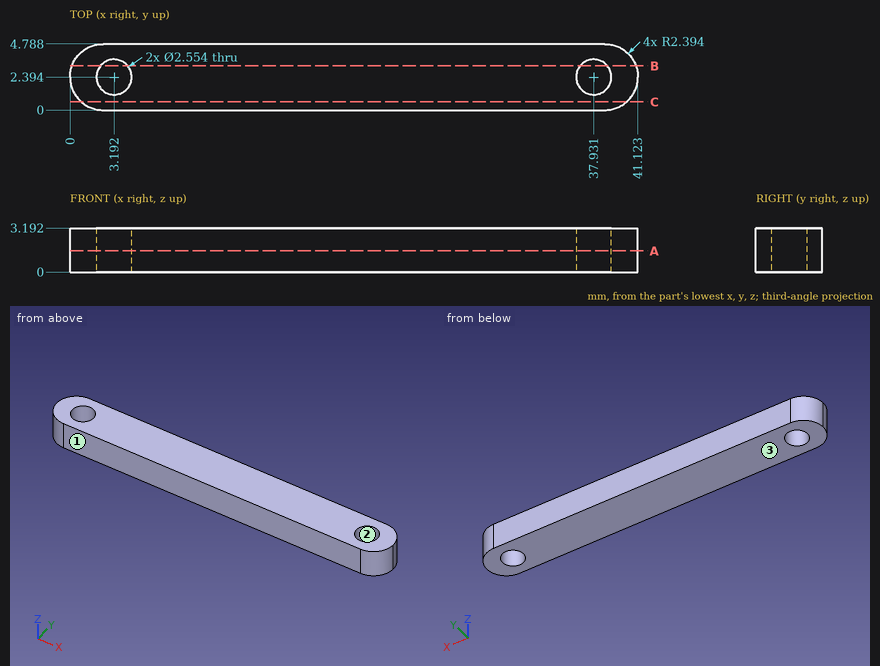
Verification items for this drawing (mm, ordinates from the low corner). Give positions to 0.01 mm unless a question says otherwise; leave off trailing zeros. Loops run counter-clockwise (first coordinate to the right, second up) from the corner with the lowest first, then second, coordinate; pieces in that order, holes last. Notation, with made-up numbers: M 84,14 L 119,14 A35 ccw 119,49 Z; hole C 59.25,20.25 d4. An arc over 180 degrees is marked long. Answer as a JSON object with one key per item and string values. Group by question number.
Q1. Material ranges on line 1 along X through (y, z) = (2.7, 2.65); line 2 along X through (y, z) = (2.6, 2.8); line 3 along Y through (x, z) = (37, 2.65) (1 decimal), recorded low to high. Write a range as [from, to].
Q2. Cross-section at A-A on z = 1.55. Give the number of separate pieces and of enclosed holes in the cut face, then the cut area to 3 significant figures.
Q3. Cross-section at B-B on y = 3.2. Record the cut outline in (x, z).
Q4. Cross-section at C-C on y = 0.6. Record the cut outline in (x, z).
Q5. Release check for a two-part mould opening along Y. For the marked faces 1, 2 and 3 record: released by +Y, released by -Y, zero draft, split by the parting line, or undercut.
Evaluation:
{
 "1": {"line 1": "x = [0.02, 1.95], [4.43, 36.69], [39.17, 41.1]", "line 2": "x = [0.01, 1.93], [4.45, 36.67], [39.19, 41.11]", "line 3": "y = [0, 1.5], [3.3, 4.8]"},
 "2": {"separate pieces": "1", "enclosed holes": "2", "area": "182 mm2"},
 "3": {"outline": "M 0.14,0 L 2.2,0 L 2.2,3.19 L 0.14,3.19 Z; M 4.18,0 L 36.94,0 L 36.94,3.19 L 4.18,3.19 Z; M 38.92,0 L 40.98,0 L 40.98,3.19 L 38.92,3.19 Z"},
 "4": {"outline": "M 0.81,0 L 40.31,0 L 40.31,3.19 L 0.81,3.19 Z"},
 "5": {"face 1": "released by -Y", "face 2": "undercut", "face 3": "zero draft"}
}
